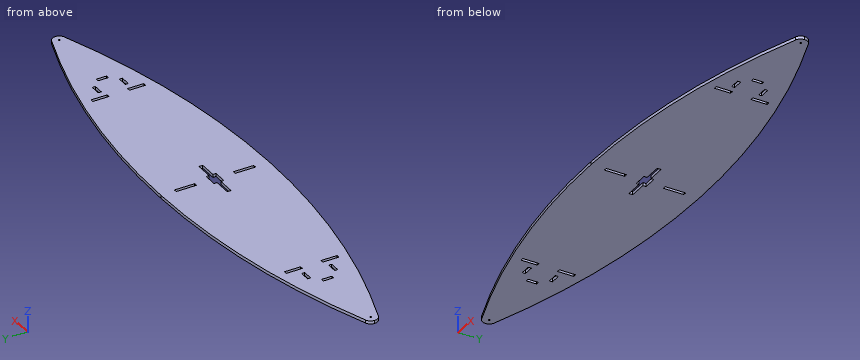
from build123d import *

# Parameters (mm, degrees)
F1_DEPTH  = 5.715
F4_DEPTH  = 5.716
F5_W      = 5.715
F5_H      = 38.1
F6_DEPTH  = 5.716
F7_W      = 5.715
F7_H      = 30.48
F8_DEPTH  = 5.716
F9_W      = 19.05
F9_H      = 5.715
F9_W_2    = 5.715
F9_H_2    = 19.05
F10_DEPTH = 5.716
F11_R     = 1.524
F12_DEPTH = 5.716


with BuildPart() as f1:
    # F0 (on Top) → F1 (new body)
    with BuildSketch(Plane.XY):
        with BuildLine():
            ThreePointArc((0, 101.6), (-253.851116, 78.999073), (-499.716688, 11.907261))
            ThreePointArc((-499.716688, 11.907261), (-505.725496, 7.252519), (-508, 0))
            ThreePointArc((-508, 0), (-505.725496, -7.252519), (-499.716688, -11.907261))
            ThreePointArc((-499.716688, -11.907261), (-253.851116, -78.999073), (0, -101.6))
            ThreePointArc((0, -101.6), (253.851116, -78.999073), (499.716688, -11.907261))
            ThreePointArc((499.716688, -11.907261), (505.725496, -7.252519), (508, 0))
            ThreePointArc((508, 0), (505.725496, 7.252519), (499.716688, 11.907261))
            ThreePointArc((499.716688, 11.907261), (253.851116, 78.999073), (0, 101.6))
        make_face()
    extrude(amount=F1_DEPTH)

    # F3 (on face) → F4 (cut, through all)
    with BuildSketch(Plane.XY.offset(5.715)):
        Polygon((-45.085, 3.556), (-45.085, 0), (-45.085, -3.556), (-12.7, -3.556), (-12.7, -9.271), (0, -9.271), (12.7, -9.271), (12.7, -3.556), (45.085, -3.556), (45.085, 0), (45.085, 3.556), (12.7, 3.556), (12.7, 9.271), (0, 9.271), (-12.7, 9.271), (-12.7, 3.556), align=None)
    extrude(amount=-F4_DEPTH, mode=Mode.SUBTRACT)

    # F5 (on face) → F6 (cut, through all)
    with BuildSketch(Plane.XY.offset(5.715)):
        with Locations((0, 55.4355)):
            Rectangle(F5_W, F5_H)
        with Locations((0, -55.4355)):
            Rectangle(F5_W, F5_H)
    extrude(amount=-F6_DEPTH, mode=Mode.SUBTRACT)

    # F7 (on face) → F8 (cut, through all)
    with BuildSketch(Plane.XY.offset(5.715)):
        with Locations((-307.6575, 34.29)):
            Rectangle(F7_W, F7_H)
        with Locations((-307.6575, -34.29)):
            Rectangle(F7_W, F7_H)
        with Locations((307.6575, -34.29)):
            Rectangle(F7_W, F7_H)
        with Locations((307.6575, 34.29)):
            Rectangle(F7_W, F7_H)
    extrude(amount=-F8_DEPTH, mode=Mode.SUBTRACT)

    # F9 (on face) → F10 (cut, through all)
    with BuildSketch(Plane.XY.offset(5.715)):
        with Locations((-332.994, 25.3365)):
            Rectangle(F9_W, F9_H)
        with Locations((-358.3305, 0)):
            Rectangle(F9_W_2, F9_H_2)
        with Locations((-332.994, -25.3365)):
            Rectangle(F9_W, F9_H)
        with Locations((332.994, -25.3365)):
            Rectangle(F9_W, F9_H)
        with Locations((358.3305, 0)):
            Rectangle(F9_W_2, F9_H_2)
        with Locations((332.994, 25.3365)):
            Rectangle(F9_W, F9_H)
    extrude(amount=-F10_DEPTH, mode=Mode.SUBTRACT)

    # F11 (on face) → F12 (cut, through all)
    with BuildSketch(Plane.XY.offset(5.715)):
        with Locations((-495.3, 0)):
            Circle(F11_R)
        with Locations((495.3, 0)):
            Circle(F11_R)
    extrude(amount=-F12_DEPTH, mode=Mode.SUBTRACT)


solid = f1.part
Geometry check sheet. Reference: the model listing, model coordinates, mm. Round coordinates to 2 decimals unless told otherwise and drop trailing zeros. Write each loop counter-clockwise with the first axis right and the second up, starting at its lowest first coordinate (ties: lowest second). Pieces come first, ordered by that corner, then holes. Notation, with made-up numbers: (81, 5) -> (87, 5) arc R25 ccw to (87, 31) -> close; hole circle Ø9 at (33, -23.75). An arc over 180 degrees is marked (long way). One line per item, written item: value. Start each with the question number.
(1) Go/stop test with flat-tipped pins: pin 1 Ø1.7 at (y, z) = (6.5, 3.5) entering from -X; pin 2 Ø3 at (x, z) = (359, 2) entering from +Y; pin 3 Ø1.7 at (x, z) = (328.5, 2.5) entering from +Y. Record where each tip stops, or that it passes through.
(2) Cross-section at B-B, the plane z = 2.9. Give the number of separate pieces and of enclosed holes in the cut face, and give its area (3 significant figures).
(3) Cross-section at A-A, the plane x = 35. Record the cut outline in (y, z) (3 decimals), and give its area (3 significant figures).
(4) Scan lines: line 1 (Y direction, x = 307.5, z = 2.65); line 2 (Y direction, x = 495.3, z = 2.8); line 3 (Y direction, x = -240, z = 4.6). Record each from-to range of solid material in increasing order. Write a range as [from, to].
Answer:
1. pin 1: x = -506.67
1. pin 2: y = 56.42
1. pin 3: y = 63.75
2. separate pieces: 1
2. enclosed holes: 15
2. area: 142,000 mm²
3. outline: (-101.174, 0) -> (-3.556, 0) -> (-3.556, 5.715) -> (-101.174, 5.715) -> close; (3.556, 0) -> (101.174, 0) -> (101.174, 5.715) -> (3.556, 5.715) -> close
3. area: 1,120 mm²
4. line 1: [-68.31, -49.53], [-19.05, 19.05], [49.53, 68.31]
4. line 2: [-13.54, -1.52], [1.52, 13.54]
4. line 3: [-81.42, 81.42]
